Autodesk Inventor part; units mm, degrees
ref_plane "Work Plane1" through (-3.0607, -16.2055, -14.9496) normal (0, 1, 0) x (0.7071068, 0, 0.7071068)
ref_plane "Work Plane2" through (-3.4749, -17.2055, -14.9496) normal (0, -1, 0) x (0.7071068, 0, -0.7071068)
ref_plane "YZ Plane" through (0, 0, 0) normal (1, 0, 0) x (0, 1, 0)
sketch "Sketch1" plane through (0, 0, 0) normal (0, 0, 1) x (1, 0, 0)
  line L0 (122.2883, -16.0055) -> (122.2883, 46.9321)
  line L1 (122.2883, -16.0055) -> (128.4096, -16.0055)
  line L2 (128.4096, -16.0055) -> (128.4096, 44.4321)
  line L3 (136.1877, 44.4321) -> (128.4096, 44.4321)
  line L4 (136.1877, 46.9321) -> (136.1877, 44.4321)
  line L5 (122.2883, 46.9321) -> (136.1877, 46.9321)
  line L6 (3.0607, 16.0055) -> (-1.0607, 16.0055)
  line L7 (122.2883, 16.0055) -> (128.4096, 16.0055)
  point P0 (0, 0)
extrude "Extrusion1" add sketch "Sketch1" against normal blind 2 contours L0 L7 L2 L1
sketch "Sketch2" plane through (122.2883, -16.0055, 0) normal (0, -1, 0) x (1, 0, 0)
  line L0 (0, 0) -> (6.1213, 0)
  line L1 (0, 0) -> (0, -2)
  line L2 (6.1213, -2) -> (0, -2)
  line L3 (6.1213, 0) -> (6.1213, -2)
  point P0 (-122.2883, 0)
ref_plane "Work Plane1" through (-3.0607, -16.2055, -14.9496) normal (0, 1, 0) x (0.7071068, 0, 0.7071068)
extrude "Extrusion2" add sketch "Sketch2" along normal up to surface (0.2 mm away)
ref_plane "Work Plane2" through (-3.4749, -17.2055, -14.9496) normal (0, -1, 0) x (0.7071068, 0, -0.7071068)
sketch "Sketch3" plane through (122.2883, -16.2055, -2) normal (0, -1, 0) x (1, 0, 0)
  line L0 (0, 2) -> (0, 0)
  line L1 (0, 0) -> (6.1213, 0)
  line L2 (6.1213, 0) -> (6.1213, 2)
  line L3 (6.1213, 2) -> (0, 2)
  arc A0 (-123.3489, 2) -> (-125.3489, 0) centre (-123.3489, 0) ccw
  line L4 (-125.3489, 0) -> (-122.3489, -3)
  line L5 (-122.3489, -3) -> (-118.1063, -3)
  line L6 (-118.1063, -3) -> (-110.278, -10.8283)
  line L7 (-110.278, -10.8283) -> (-110.278, 0)
  line L8 (-110.278, 0) -> (-114.7423, 0)
  line L9 (-114.7423, 0) -> (-114.9849, 0.2426)
  arc A1 (-114.9849, 0.2426) -> (-119.2276, 2) centre (-119.2276, -4) ccw
  line L10 (-119.2276, 2) -> (-123.3489, 2)
  line L11 (-110.278, -10.8283) -> (8.4603, -10.8283)
  line L12 (-110.278, -10.8283) -> (8.4603, -10.8283) construction
  arc A2 (0, 0) -> (-2.8284, -1.1716) centre (0, -4) ccw
  line L13 (-54.1499, -52.493) -> (-2.8284, -1.1716)
  line L14 (-12.4852, -10.8283) -> (-1.6569, -10.8283) construction
  arc A3 (0, 2) -> (-4.2426, 0.2426) centre (0, -4) ccw
  line L15 (-1.1213, -3) -> (-18.8648, -20.7435)
  line L16 (3.1213, -3) -> (-1.1213, -3)
  line L17 (6.1213, 0) -> (3.1213, -3)
  line L18 (-8.9496, -10.8283) -> (81.0504, -10.8283) construction
  line L19 (-8.9496, -10.8283) -> (-8.9496, 0)
  line L20 (-8.9496, -10.8283) -> (1.8787, -10.8283) construction
  line L21 (-8.9496, 0) -> (-4.4853, 0)
  line L22 (-55.5641, -51.0788) -> (-8.9496, -4.4643)
  line L23 (-4.4853, 0) -> (-4.2426, 0.2426)
  point P0 (-122.2883, 2)
extrude "Extrusion3" add sketch "Sketch3" along normal up to surface (1 mm away) contours L3 L2 L1 L0 | L0 A2 L13 L19 L21 L23 A3 | L1 L17 L16 L15 L19 L13 A2
sketch "Sketch4" plane through (122.2883, -16.2055, -2) normal (0, 1, 0) x (1, 0, 0)
  line L0 (-2.8284, 1.1716) -> (-33.605, 31.9482)
  arc A0 (-2.8284, 1.1716) -> (0, 0) centre (0, 4) ccw
  line L1 (0, -2) -> (0, 0)
  arc A1 (-4.2426, -0.2426) -> (0, -2) centre (0, 4) ccw
  line L2 (-4.2426, -0.2426) -> (-4.4853, 0)
  line L3 (-4.4853, 0) -> (-8.9496, 0)
  line L4 (-8.9496, 0) -> (-8.9496, 10.8283)
  point P0 (-122.2883, -2)
  point P1 (-8.9496, 7.2928)
extrude "Extrusion4" add sketch "Sketch4" along normal up to surface (32.211 mm away)
fillet "Fillet1" radius 2 1 edges at (128.4096, -0.6, 0)
sketch "Sketch6" plane through (113.3386, -17.2055, -2) normal (-1, 0, 0) x (0, 0, 1)
  circle A0 centre (6.5566, 27.211) radius 35
  line L0 (-7.2928, 1) -> (-7.2928, 33.211)
  line L1 (-10.8283, 0) -> (0, 0)
  line L2 (0, 33.211) -> (0, 0)
  line L3 (0, 33.211) -> (-7.2928, 33.211)
  line L4 (-7.2928, 1) -> (-7.2928, 33.211)
  line L5 (-7.2928, 1) -> (-10.8283, 1)
  line L6 (-10.8283, 1) -> (-10.8283, 0)
  line L7 (0, 27.211) -> (-7.2928, 27.211)
  circle A1 centre (-3.6464, 27.211) radius 2.5
  point P0 (2, 17.2055)
  dimension "d16" = 5
extrude "Extrusion5" add sketch "Sketch6" along normal blind 4 contours A1 L7 | L7 A1
chamfer "Chamfer1" distance 0.5 angle 45 1 edges at (113.3386, 10.0055, -8.1464)
sketch "Sketch7" plane through (109.3386, 10.0055, -5.6464) normal (-1, 0, 0) x (0, 0, 1)
  circle A0 centre (0, 0) radius 2.5
  circle A1 centre (0, 0) radius 1.5
  point P0 (5.6464, -10.0055)
  dimension "d22" = 3
extrude "Extrusion6" cut sketch "Sketch7" against normal through all contours A1
sketch "Sketch8" plane through (0, 0, 0) normal (0, 0, 1) x (1, 0, 0)
  line L0 (126.4096, 16.0055) -> (126.4096, -17.2055)
  line L1 (126.4096, 16.0055) -> (122.2883, 16.0055)
  line L2 (122.2883, 16.0055) -> (122.2883, -17.2055)
  line L3 (122.2883, -17.2055) -> (126.4096, -17.2055)
  line L4 (122.2883, 16.0055) -> (119.4598, 16.0055)
  line L5 (122.2883, 16.0055) -> (126.4096, 16.0055)
  line L6 (126.4096, 16.0055) -> (126.4096, 12.0055)
  line L7 (126.4096, 12.0055) -> (122.2883, 12.0055)
  line L8 (122.2883, 12.0055) -> (122.2883, 16.0055)
  line L9 (122.2883, -17.2055) -> (126.4096, -17.2055)
  line L10 (126.4096, -17.2055) -> (126.4096, -13.2055)
  line L11 (126.4096, -13.2055) -> (122.2883, -13.2055)
  line L12 (122.2883, -13.2055) -> (122.2883, -17.2055)
  circle A0 centre (124.3489, 9.9448) radius 2.0607
  circle A1 centre (124.3489, -11.1448) radius 2.0607
  circle A2 centre (124.3489, 9.9448) radius 1.5
  circle A3 centre (124.3489, -11.1448) radius 1.5
  point P0 (0, 0)
  dimension "d25" = 4
  dimension "d26" = 4
  dimension "d27" = 3
  dimension "d28" = 3
extrude "Extrusion7" cut sketch "Sketch8" against normal blind 10 contours A2 | A3
properties part number "GripperHandleLeft_3DPrint"
Input: part model. Units: mm. Frame: model coordinates. A direction names the side the tool comes from. Coordinates: 2 decimals unless noted, no trailing zeros. Write each loop counter-clockwise with the first axis right and the second up, starting at its lowest first coordinate (ties: lowest second). Pieces come first, ordered by that corner, then holes. Notation, with made-up numbers: (-17.5, -4) -> (41.5, -4) arc R31 cw to (41.5, 25) -> close; hole circle Ø9 at (-38.75, -16). An arc over 180 degrees is marked (long way). Answer as a JSON object with one key per item and string values.
1. Mould query, pull axis Z, two halves, no side actions, for faces 5 (the face through (120.023, -0.325, -0.444)), 6 (the face through (119, -17.206, -5)), 7 (the face through (112.832, 10.456, -4.216)). Classes: released by +Z, released by -Z, zero draft, split by the parting line, or undercut.
Result set:
{"face 5": "released by +Z", "face 6": "zero draft", "face 7": "undercut"}
2. Access query for faces 1 (the face through (120.778, -0.325, -2.296)), 2 (the face through (123, -17, -5)), 3 (the face through (116, -1, -2)), 4 (the face through (111.113, 9.896, -8.144)). Directions: +Z, -Z, +X, -X, +Y, -Y. A direction counts if a zero-diameter tool reaches every point of the face in a straight line with its end or side. Return the directions, or none.
Result set:
{"face 1": "-Z, +X, +Y", "face 2": "-Z, +X, +Y, -Y", "face 3": "+Z, -X, +Y, -Y", "face 4": "-X"}
3. Section A-A on x = 123.5. Return the cut outline in (y, z), then the cut area to 3 significant figures.
Result set:
{"outline": "(-17.21, -5) -> (-16.21, -5) -> (-16.21, -2) -> (-12.38, -2) -> (-12.38, 0) -> (-17.21, 0) -> close; (-9.91, -2) -> (8.71, -2) -> (8.71, 0) -> (-9.91, 0) -> close; (11.18, -2) -> (16.01, -2) -> (16.01, 0) -> (11.18, 0) -> close", "area": "59.5 mm2"}
4. First-contact query: P1, Ø2, axis at x = 117, y = -6.5, coming from the +Z side; P2, Ø1.8, axis at x = 125.5, y = 1.5, coming from the -Z side; P3, Ø5, axis at x = 116.5, y = 0.5, coming from the +Z side. Flat tips, straight axial feed; report the tip coordinate or a pass-through.
Result set:
{"P1": "stops at z = -1.8", "P2": "stops at z = -2", "P3": "stops at z = -0.98"}
5. Section C-C on x = 120.5. Return the cut outline in (y, z), then the cut area to 3 significant figures.
Result set:
{"outline": "(-17.21, -5.67) -> (-16.21, -5.67) -> (-16.21, -2.42) -> (16.01, -2.42) -> (16.01, -0.27) -> (-17.21, -0.27) -> close", "area": "74.6 mm2"}
6. Material intervals for line 1 (Y direction, x = 112.5, z = -5.75); line 2 (Z direction, x = 125, y = 8.5); line 3 (Y direction, x = 115.5, z = -10.5), sorted ascending. Write a range as from..to.
Result set:
{"line 1": "y = 7.51..8.51, 11.5..12.5", "line 2": "z = -2..0", "line 3": "y = -17.21..-16.21"}
7. Section D-D on x = 111. Return the cut outline in (y, z).
Result set:
{"outline": "circle Ø5 at (10.01, -5.65); hole circle Ø3 at (10.01, -5.65)"}
